Check sheet for the modelled part. Datum: model origin and axes. Units: mm. Round coordinates to 2 decimals unless told otherwise and drop trailing zeros. Write each loop counter-clockwise with the first axis right and the second up, starting at its lowest first coordinate (ties: lowest second). Pieces come first, ordered by that corner, then holes. Notation, with made-up numbers: (20.5, -17.75) -> (74.5, -17.75) arc R27 ccw to (74.5, 9.25) -> close; hole circle Ø6 at (-29, 62.5). An arc over 180 degrees is marked (long way). One line per item, written item: value.
from build123d import *

# Parameters (mm, degrees)
SKETCH1_W           = 32.13640153
SKETCH1_H           = 27.772655408
SKETCH1_R           = 3
SKETCH1_R_2         = 1.75
BOSS_EXTRUDE1_DEPTH = 1


with BuildPart() as part:
    # Sketch1 → Boss-Extrude1 (new, symmetric)
    # profile 1 of 5: a face of its own
    with BuildSketch(Plane(origin=(0, 0, 0), x_dir=(-0.9848077530122068, -0.17364817766693766, 0), z_dir=(0, 0, 1))):
        Rectangle(SKETCH1_W, SKETCH1_H)
        with Locations((0, -9.5)):
            Circle(SKETCH1_R, mode=Mode.SUBTRACT)
        with Locations((12.5, 0)):
            Circle(SKETCH1_R, mode=Mode.SUBTRACT)
        with Locations((0, 9.5)):
            Circle(SKETCH1_R, mode=Mode.SUBTRACT)
        with Locations((-12.5, 0)):
            Circle(SKETCH1_R, mode=Mode.SUBTRACT)
    # profile 2 of 5: a face of its own
    with BuildSketch(Plane(origin=(0, 0, 0), x_dir=(-0.9848077530122068, -0.17364817766693766, 0), z_dir=(0, 0, 1))):
        with Locations((-12.5, 0)):
            Circle(SKETCH1_R)
        with Locations(Location((-12.5, 0, 0), (0, 0, 170))):
            Circle(SKETCH1_R_2, mode=Mode.SUBTRACT)
    # profile 3 of 5: a face of its own
    with BuildSketch(Plane(origin=(0, 0, 0), x_dir=(-0.9848077530122068, -0.17364817766693766, 0), z_dir=(0, 0, 1))):
        with Locations((0, -9.5)):
            Circle(SKETCH1_R)
        with Locations(Location((0, -9.5, 0), (0, 0, 170))):
            Circle(SKETCH1_R_2, mode=Mode.SUBTRACT)
    # profile 4 of 5: a face of its own
    with BuildSketch(Plane(origin=(0, 0, 0), x_dir=(-0.9848077530122068, -0.17364817766693766, 0), z_dir=(0, 0, 1))):
        with Locations((0, 9.5)):
            Circle(SKETCH1_R)
        with Locations(Location((0, 9.5, 0), (0, 0, 170))):
            Circle(SKETCH1_R_2, mode=Mode.SUBTRACT)
    # profile 5 of 5: a face of its own
    with BuildSketch(Plane(origin=(0, 0, 0), x_dir=(-0.9848077530122068, -0.17364817766693766, 0), z_dir=(0, 0, 1))):
        with Locations((12.5, 0)):
            Circle(SKETCH1_R)
        with Locations(Location((12.5, 0, 0), (0, 0, 170))):
            Circle(SKETCH1_R_2, mode=Mode.SUBTRACT)
    extrude(amount=BOSS_EXTRUDE1_DEPTH, both=True)


solid = part.part
Item 1: Sectioned sample at A-A (y = 8). Enter the section's corners in (x, z), then the cut area to 3 significant figures.
Result set:
outline: (-17.73, -1) -> (-2.76, -1) -> (-2.76, 1) -> (-17.73, 1) -> close; (-0.54, -1) -> (14.91, -1) -> (14.91, 1) -> (-0.54, 1) -> close
area: 60.8 mm^2
Item 2: Sectioned sample at B-B (z = -0.5). Enter the section's corners in (x, y), then the cut area to 3 significant figures.
Result set:
outline: (-18.24, 10.89) -> (-13.41, -16.47) -> (18.24, -10.89) -> (13.41, 16.47) -> close; hole circle Ø3.5 at (-12.31, -2.17); hole circle Ø3.5 at (-1.65, 9.36); hole circle Ø3.5 at (1.65, -9.36); hole circle Ø3.5 at (12.31, 2.17)
area: 854 mm^2
Item 3: Sectioned sample at C-C (x = -3). Enter the section's corners in (y, z), then the cut area to 3 significant figures.
Result set:
outline: (-14.63, -1) -> (8.24, -1) -> (8.24, 1) -> (-14.63, 1) -> close; (10.47, -1) -> (13.57, -1) -> (13.57, 1) -> (10.47, 1) -> close
area: 51.9 mm^2
Item 4: Depth check by flat-ended pin: pin 1 (2 mm diameter, centred on x = 12.31, y = 2.17, fed in from -Z). Enter the tip coordinate at first touch or a pass-through.
Result set:
pin 1: through
Item 5: Material ranges on line 1 along X through (y, z) = (-10, 0.7); line 2 along X through (y, z) = (1.5, -0.05); line 3 along Y through (x, z) = (11, 0.8), recorded low to high.
Result set:
line 1: -14.55 to 0.02, 3.28 to 18.08
line 2: -16.58 to 10.69, 13.93 to 16.05
line 3: -12.16 to 1.01, 3.33 to 16.04
